Geometry: final body of the model. Coordinates: model frame, mm. Face numbers are marked on the shaded views. A direction names the side the tool comes from. Coordinates: 2 decimals unless noted, no trailing zeros. Write each loop counter-clockwise with the first axis right and the second up, starting at its lowest first coordinate (ties: lowest second). Pieces come first, ordered by that corner, then holes.
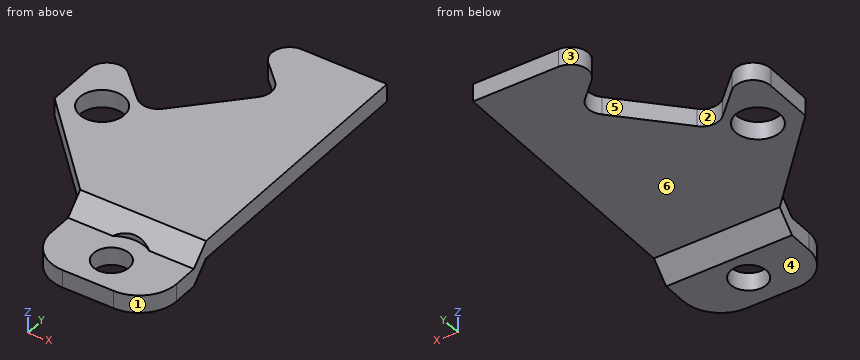
Autodesk Inventor part; units mm, degrees
ref_plane "YZ Plane" through (0, 0, 0) normal (1, 0, 0) x (0, 1, 0)
ref_plane "XZ Plane" through (0, 0, 0) normal (0, 1, 0) x (-1, 0, 0)
ref_plane "XY Plane" through (0, 0, 0) normal (0, 0, 1) x (1, 0, 0)
sketch "Sketch1" plane through (0, 0, 0) normal (0, 0, 1) x (1, 0, 0)
  circle A0 centre (0, 0) radius 1.25
  line L0 (-4.75, 9.95) -> (2.5, 9.95)
  line L1 (2.5, 9.95) -> (2.5, -4.95)
  line L2 (2.5, -4.95) -> (-4.75, -4.95)
  line L3 (-4.75, -4.95) -> (-4.75, 9.95)
  line L4 (-4.75, 4.85) -> (-9.65, 4.85)
  line L5 (-9.65, 4.85) -> (-9.65, 0.15)
  line L6 (-9.65, 0.15) -> (-4.75, 0.15)
  line L7 (-4.75, 0.15) -> (-4.75, 4.85)
  line L8 (-4.75, -4.95) -> (-9.65, 0.15)
  line L9 (-9.65, 4.85) -> (-4.75, 9.95)
  line L10 (-9.65, 4.85) -> (-13.2555, 8.3141)
  line L11 (-4.75, 9.95) -> (-8.2862, 13.4862)
  line L12 (-13.2555, 8.3141) -> (-8.2862, 13.4862)
  circle A1 centre (-7.5, 1) radius 1.25
  line L13 (-9.5461, 4.9582) -> (-13.1516, 8.4223)
  line L14 (-4.8539, 9.8418) -> (-8.3902, 13.3781)
  line L15 (2.4, 9.95) -> (2.4, -4.95)
  line L16 (-9.65, 0.2541) -> (-4.65, -4.95)
  point P0 (-8.4165, 0.15)
  point P1 (-6.5835, 0.15)
  point P2 (-9.55, 0.15)
  point P3 (-4.75, -4.8459)
  dimension "d26" = 4.95
  dimension "d27" = 7.25
  dimension "d28" = 2.5
  dimension "d29" = 4.9
  dimension "d30" = 14.9
  dimension "d31" = 5.1
  dimension "d32" = 5.1
  dimension "d33" = 90
  dimension "d34" = 135
  dimension "d36" = 0
  dimension "d37" = 0
  dimension "d38" = 2.5
  dimension "d39" = 5
  dimension "d40" = 2.5
  dimension "d41" = 1
  dimension "d42" = 7.5
  dimension "d43" = 0.15
  dimension "d44" = 0.15
  dimension "d54" = 0.1
  dimension "d55" = 0.1
extrude "Extrusion1" add sketch "Sketch1" along normal blind 1 contours A0 | L0 L15 L2 L16 L3 | L3 L4 L9 | L3 L6 A1 L16 L5 L4 | L3 L16 L6 A1
sketch "Sketch7" plane through (0, 0, 0) normal (0, 0, -1) x (-1, 0, 0)
  line L0 (4.65, -4.95) -> (-2.4, -4.95)
  line L1 (9.65, 0.2541) -> (4.65, -4.95)
  line L2 (9.65, 4.85) -> (9.65, 0.2541)
  line L3 (4.75, 9.95) -> (9.65, 4.85)
  line L4 (-2.4, 9.95) -> (4.75, 9.95)
  line L5 (-2.4, -4.95) -> (-2.4, 9.95)
  circle A0 centre (7.5, 1) radius 1.25
  line L6 (4.65, -4.95) -> (-2.4, -4.95)
  line L7 (-2.4, -4.95) -> (4.65, -4.95)
  line L8 (4.65, -4.95) -> (4.65, -9.45)
  line L9 (4.65, -9.45) -> (-2.4, -9.45)
  line L10 (-2.4, -9.45) -> (-2.4, -4.95)
  circle A1 centre (1.125, -7.55) radius 1
  line L11 (4.75, 9.95) -> (8.2855, 13.4855)
  line L12 (4.75, 9.95) -> (9.75, 9.95) construction
  line L13 (9.65, 4.85) -> (13.1855, 8.3855)
  line L14 (9.65, 4.85) -> (14.65, 4.85) construction
  line L15 (13.1855, 8.3855) -> (8.2855, 13.4855)
  line L16 (9.5114, 4.9942) -> (13.0469, 8.5298)
  line L17 (-2.4, -4.95) -> (-2.4, 9.95)
  line L18 (-2.4, 9.85) -> (4.8461, 9.85)
  line L19 (4.8461, 9.85) -> (8.3816, 13.3855)
  point P0 (0, 0)
  dimension "d56" = 0
  dimension "d57" = 4.5
  dimension "d58" = 2
  dimension "d59" = 3.525
  dimension "d60" = 2.6
  dimension "d63" = 5
  dimension "d64" = 45
  dimension "d65" = 5
  dimension "d66" = 45
  dimension "d68" = 0.2
  dimension "d69" = 0.1
extrude "Extrusion5" add sketch "Sketch7" against normal mid plane 2 contours L8 L9 L10 L0 | L19 L15 L16 L3
fillet "Fillet2" radius 2.1 2 edges at (-4.65, -9.45, 0) (2.4, -9.45, 0)
sketch "Sketch8" plane through (0, 0, 1) normal (0, 0, 1) x (1, 0, 0)
  line L0 (2.4, 9.95) -> (-4.75, 9.95)
  line L1 (-4.75, 9.95) -> (-4.8461, 9.85)
  line L2 (2.4, -7.35) -> (2.4, 9.95)
  line L3 (-4.75, 9.95) -> (-4.8461, 9.85)
  line L4 (-4.8461, 9.85) -> (2.4, 9.85)
  point P0 (0, 0)
extrude "Extrusion6" cut sketch "Sketch8" against normal up to surface (1 mm away)
chamfer "Chamfer1" distance 1 angle 45 2 edges at (-1.125, -4.95, -1) (-7.1787, 7.4221, -1)
sketch "Sketch9" plane through (0, 0, 1) normal (0, 0, 1) x (1, 0, 0)
  line L0 (-4.65, -4.95) -> (2.4, -4.95)
  line L1 (2.4, -5.95) -> (-4.65, -5.95)
  line L2 (2.4, 9.85) -> (-4.8461, 9.85)
  line L3 (-4.8461, 9.85) -> (-8.3816, 13.3855)
  line L4 (-8.3816, 13.3855) -> (-13.0469, 8.5298)
  line L5 (-13.0469, 8.5298) -> (-9.5114, 4.9942)
  line L6 (-9.5114, 4.9942) -> (-9.65, 4.85)
  line L7 (-9.65, 4.85) -> (-9.65, 0.2541)
  line L8 (-9.65, 0.2541) -> (-4.65, -4.95)
  line L9 (-4.65, -4.95) -> (-4.65, -7.35)
  arc A0 (-4.65, -7.35) -> (-2.55, -9.45) centre (-2.55, -7.35) ccw
  line L10 (-2.55, -9.45) -> (0.3, -9.45)
  arc A1 (0.3, -9.45) -> (2.4, -7.35) centre (0.3, -7.35) ccw
  line L11 (2.4, -7.35) -> (2.4, 9.85)
  circle A2 centre (-1.125, -7.55) radius 1
  circle A3 centre (-7.5, 1) radius 1.25
  point P0 (0, 0)
extrude "Extrusion7" cut sketch "Sketch9" against normal blind 1 contours L1 L11 A1 L10 A0 L9
chamfer "Chamfer2" distance 1 angle 45 1 edges at (-1.125, -5.95, 1)
sketch "Sketch10" plane through (0, 0, 0) normal (0, 0, 1) x (1, 0, 0)
  circle A0 centre (-1.125, -7.55) radius 1
  circle A1 centre (-1.125, -7.55) radius 1.9
  point P0 (0, 0)
  dimension "d80" = 3.8
extrude "Extrusion8" cut sketch "Sketch10" along normal up to surface (1 mm away)
sketch "Sketch11" plane through (0, 0, 1) normal (0, 0, 1) x (1, 0, 0)
  line L0 (-6.2966, 11.2255) -> (-10.8, 6.5383)
  line L1 (-10.8, 6.5383) -> (-5.7523, 1.6886)
  line L2 (-5.7523, 1.6886) -> (-1.2489, 6.3757)
  line L3 (-1.2489, 6.3757) -> (-6.2966, 11.2255)
  line L4 (-6.2966, 11.2255) -> (-5.7523, 1.6886) construction
  line L5 (-10.8, 6.5383) -> (-1.2489, 6.3757) construction
  line L6 (-8.3816, 13.3855) -> (-13.0469, 8.5298)
  line L7 (-13.0469, 8.5298) -> (-9.5114, 4.9942)
  line L8 (-4.8461, 9.85) -> (-8.3816, 13.3855)
  line L9 (-4.8461, 9.85) -> (2.4, 9.85)
  line L10 (-4.8461, 9.85) -> (-4.8551, 9.8406)
  line L11 (-4.8461, 9.85) -> (-9.5114, 4.9942)
  point P0 (0, 0)
  point P1 (-6.0245, 6.457)
  point P2 (-10.9252, 6.408)
  point P3 (-6.2599, 11.2638)
  point P4 (-9.3585, 5.1534)
  dimension "d83" = 7
  dimension "d85" = 6.5
  dimension "d86" = 3.5
  dimension "d89" = 6.5
extrude "Extrusion9" cut sketch "Sketch11" against normal up to surface (2 mm away)
fillet "Fillet3" radius 1 1 edges at (-5.7523, 1.6886, 0.5)
fillet "Fillet4" radius 1 5 edges at (-9.3585, 5.1534, 0.5) (-9.65, 4.85, 0.5) (-1.2489, 6.3757, 0.5) (-4.8551, 9.8406, 0.5) (-4.8461, 9.85, 0.5)
Item 1: Section C-C, the plane z = -0.5. Output: boundary loops of the cut face in (x, y) (3 decimals).
Derived:
outline: (-4.65, -7.35) arc R2.1 ccw to (-2.55, -9.45) - (0.3, -9.45) arc R2.1 ccw to (2.4, -7.35) - (2.4, -5.45) - (-4.65, -5.45) - close; hole circle Ø2 at (-1.125, -7.55)
Item 2: Section B-B, the plane x = -7.5. Output: boundary loops of the cut face in (y, z), plus the area to 3 significant figures.
Derived:
outline: (-1.98, 0) - (-0.25, 0) - (-0.25, 1) - (-1.98, 1) - close; (2.25, 0) - (3.37, 0) - (3.37, 1) - (2.25, 1) - close
area: 2.85 mm2
Item 3: Section A-A, the plane y = 1. Output: boundary loops of the cut face in (x, z), plus the area to 3 significant figures.
Derived:
outline: (-9.65, 0) - (-8.75, 0) - (-8.75, 1) - (-9.65, 1) - close; (-6.25, 0) - (2.4, 0) - (2.4, 1) - (-6.25, 1) - close
area: 9.55 mm2
Item 4: Pin query (flat end, axial travel): pin 1 (1 mm diameter, centred on y = -6, z = -0.5, fed in from -X); pin 2 (1 mm diameter, centred on x = 0, y = 4.5, fed in from -Z); pin 3 (2.5 mm diameter, centred on x = -1.125, y = -7.55, fed in from +Z); pin 4 (1 mm diameter, centred on x = -4.5, y = 4.5, fed in from -Z) (3 decimals). Return the tip coordinate at first contact, or that it passes through.
Derived:
pin 1: stops at x = -4.65
pin 2: stops at z = 0
pin 3: stops at z = 0
pin 4: passes through
Item 5: Pull-direction query (X, two-part tool) for the marked faces 1, 2 and 3; classes: released by +X, released by -X, zero draft, split by the parting line, or undercut.
Derived:
face 1: released by +X
face 2: undercut
face 3: released by -X
Item 6: Material intervals for probe 1 along Z at (x, y) = (0, -4); probe 2 along X at (y, z) = (1, 0.4); probe 3 along Z at (x, y) = (-4.5, -7.25), sorted ascending.
Derived:
probe 1: z = 0 to 1
probe 2: x = -9.65 to -8.75, -6.25 to 2.4
probe 3: z = -1 to 0
Item 7: Set-up query: the marked faces 4, 5 and 6. Return all of +Z, -Z, +X, -X, +Y, -Y with unobstructed straight access to the full face (end or side cutting, diameter ignored); none if empty.
Derived:
face 4: -Z, +X, -X, +Y, -Y
face 5: +Z, -Z
face 6: -Z, +X, -X, +Y
